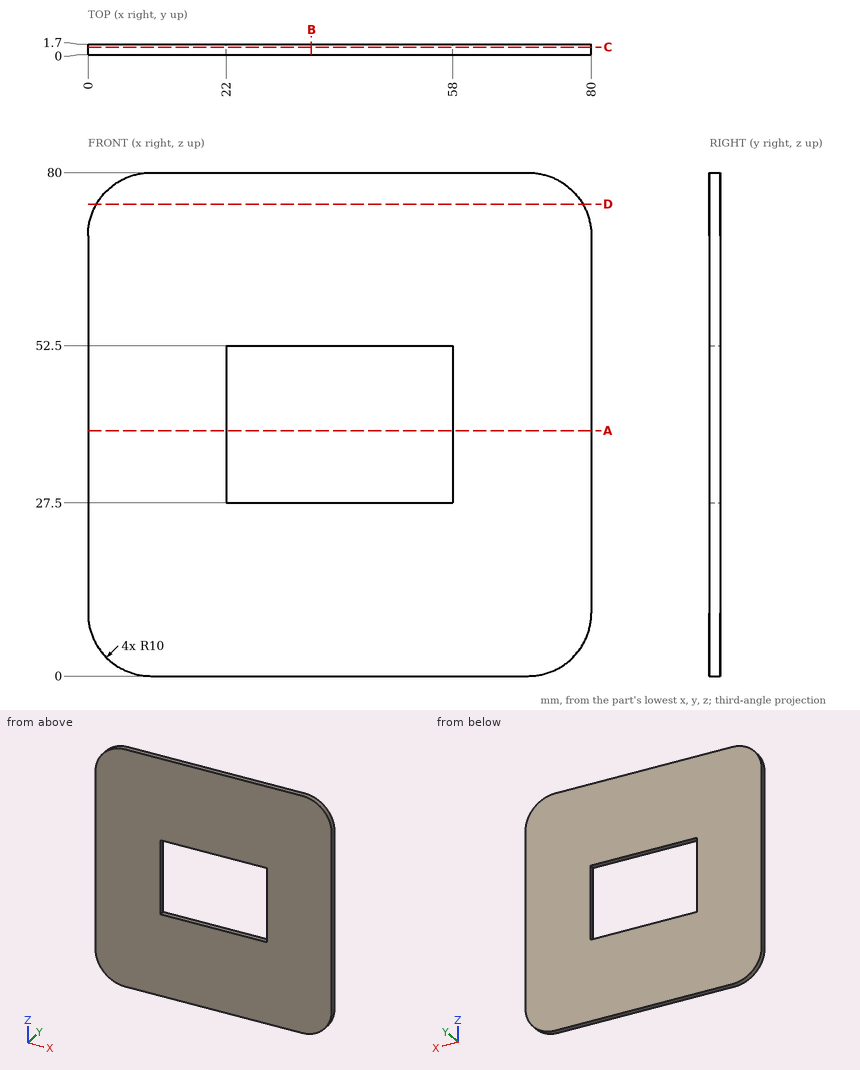
Design review of the part shown in the three views and the two pictorial views. Dimensions are in mm from the part's minimum x, y and z. Round coordinates to 2 decimals unless told otherwise and drop trailing zeros. Write each loop counter-clockwise with the first axis right and the second up, starting at its lowest first coordinate (ties: lowest second). Pieces come first, ordered by that corner, then holes. Notation, with made-up numbers: M 50,65.5 L 74,65.5 A19 cw 74,73.5 Z; hole C -10.75,64.5 d11. An arc over 180 degrees is marked long. Use a Markdown table: item, result. Add a question column.
Q1. We need section D-D, the plane z = 75. State the section outline as (x, y) points.
Q2. We need section B-B, the plane x = 35.5. State the section outline as (y, z) points, plus the area to 3 significant figures.
Q3. We need section A-A, the plane z = 39. State the section outline as (x, y) points, plus the area to 3 significant figures.
Q4. We need section C-C, the plane y = 1.2. State the section outline as (x, z) points, plus the area to 3 significant figures.
Q5. To check wall thickness, follow line 1 (Z direction, x = 36.5, y = 0.15); line 2 (X direction, y = 0.95, z = 41); line 3 (X direction, y = 0.9, z = 75). State the ranges of each line that lie inside material, in increasing order.
Findings below:
| question | item | result |
|---|---|---|
| 1 | outline | M 1.34,0 L 78.66,0 L 78.66,1.7 L 1.34,1.7 Z |
| 2 | outline | M 0,0 L 1.7,0 L 1.7,27.5 L 0,27.5 Z; M 0,52.5 L 1.7,52.5 L 1.7,80 L 0,80 Z |
| 2 | area | 93.5 mm² |
| 3 | outline | M 0,0 L 22,0 L 22,1.7 L 0,1.7 Z; M 58,0 L 80,0 L 80,1.7 L 58,1.7 Z |
| 3 | area | 74.8 mm² |
| 4 | outline | M 0,10 A10 ccw 10,0 L 70,0 A10 ccw 80,10 L 80,70 A10 ccw 70,80 L 10,80 A10 ccw 0,70 Z; hole M 22,27.5 L 58,27.5 L 58,52.5 L 22,52.5 Z |
| 4 | area | 5,410 mm² |
| 5 | line 1 | z = 0 to 27.5, 52.5 to 80 |
| 5 | line 2 | x = 0 to 22, 58 to 80 |
| 5 | line 3 | x = 1.34 to 78.66 |
